Source: CAD feature listing. Evaluate the final solid. Frame: model axes, mm. A direction names the side the tool comes from. Give positions to 0.01 mm unless a question says otherwise; leave off trailing zeros. Write each loop counter-clockwise with the first axis right and the second up, starting at its lowest first coordinate (ties: lowest second). Pieces come first, ordered by that corner, then holes. Notation, with made-up numbers: (14.5, 40.25) -> (25.5, 40.25) arc R25 ccw to (25.5, 63.25) -> close; hole circle Ø1 at (47, 64.25). An arc over 180 degrees is marked (long way). Write item = value, one per line.
from build123d import *

# Parameters (mm, degrees)
F0_W     = 215
F0_H     = 50
F1_DEPTH = 57
F3_DEPTH = 18
F4_W     = 26
F4_H     = 3
F5_DEPTH = 10


with BuildPart() as f1:
    # F0 (on Right) → F1 (new body, symmetric)
    with BuildSketch(Plane.YZ):
        with Locations((-107.5, 25)):
            Rectangle(F0_W, F0_H)
    extrude(amount=F1_DEPTH, both=True)

    # F2 (on face) → F3 (cut)
    with BuildSketch(Plane.XZ.offset(215)):
        Polygon((-55, 50), (-55, 6), (-37, 6), (-37, 21), (50, 21), (50, 6), (55, 6), (55, 50), align=None)
    extrude(amount=-F3_DEPTH, mode=Mode.SUBTRACT)

    # F4 (on face) → F5 (cut)
    with BuildSketch(Plane.XY.offset(50)):
        with Locations((22, -168.5)):
            Rectangle(F4_W, F4_H)
        with Locations((22, -172.5)):
            Rectangle(F4_W, F4_H)
        with Locations((22, -176.5)):
            Rectangle(F4_W, F4_H)
        with Locations((22, -180.5)):
            Rectangle(F4_W, F4_H)
        with Locations((22, -184.5)):
            Rectangle(F4_W, F4_H)
        with Locations((-22, -184.5)):
            Rectangle(F4_W, F4_H)
        with Locations((-22, -180.5)):
            Rectangle(F4_W, F4_H)
        with Locations((-22, -176.5)):
            Rectangle(F4_W, F4_H)
        with Locations((-22, -172.5)):
            Rectangle(F4_W, F4_H)
        with Locations((-22, -168.5)):
            Rectangle(F4_W, F4_H)
    extrude(amount=-F5_DEPTH, mode=Mode.SUBTRACT)


solid = f1.part
(1) Section query A-A (z = 29). Return loops of the section in (x, y).
Values follow:
outline = (-57, -215) -> (-55, -215) -> (-55, -197) -> (55, -197) -> (55, -215) -> (57, -215) -> (57, 0) -> (-57, 0) -> close
(2) Section query B-B (x = 0). Return loops of the section in (y, z), plus the area to 3 significant figures.
Values follow:
outline = (-215, 0) -> (0, 0) -> (0, 50) -> (-197, 50) -> (-197, 21) -> (-215, 21) -> close
area = 10,200 mm2
(3) First-contact query: pin 1 (8 mm diameter, centred on x = 18.5, z = 44.5, fed in from -Y); pin 2 (1.5 mm diameter, centred on x = 17.5, y = -176, fed in from +Z). Flat tips, straight axial feed; report the tip coordinate or a pass-through.
Values follow:
pin_1 = -197
pin_2 = 40
(4) Section query C-C (z = 46). Give the number of separate pieces and of enclosed holes in the cut face, plus the area to 4 significant figures.
Values follow:
separate_pieces = 1
enclosed_holes = 10
area = 21,750 mm2
(5) Material intervals for line 1 (Y direction, x = -27, z = 41); line 2 (Z direction, x = 28, y = -199); line 3 (Y direction, x = -40, z = 29), sorted ascending.
Values follow:
line_1 = -197 to -186, -183 to -182, -179 to -178, -175 to -174, -171 to -170, -167 to 0
line_2 = 0 to 21
line_3 = -197 to 0
(6) Section query D-D (x = 23.5). Return loops of the section in (y, z), plus the area to 3 significant figures.
Values follow:
outline = (-215, 0) -> (0, 0) -> (0, 50) -> (-167, 50) -> (-167, 40) -> (-170, 40) -> (-170, 50) -> (-171, 50) -> (-171, 40) -> (-174, 40) -> (-174, 50) -> (-175, 50) -> (-175, 40) -> (-178, 40) -> (-178, 50) -> (-179, 50) -> (-179, 40) -> (-182, 40) -> (-182, 50) -> (-183, 50) -> (-183, 40) -> (-186, 40) -> (-186, 50) -> (-197, 50) -> (-197, 21) -> (-215, 21) -> close
area = 10,100 mm2
(7) Pull-direction query (Y, two-part tool) for faces 3 (the face through (-57, -109, 25)), 4 (the face through (22, -174, 45)), 5 (the face through (1, 0, 25)); classes: pulls with the +Y half, pulls with the -Y half, needs draft (parallel to the pull), parting line crosses it, or undercut.
Values follow:
face_3 = needs draft
face_4 = undercut
face_5 = pulls with the +Y half
(8) Access query for faces 1 (the face through (55, -206, 28)), 2 (the face through (-22, -174, 45)). Directions: +Z, -Z, +X, -X, +Y, -Y. A direction counts if a zero-diameter tool reaches every point of the face in a straight line with its end or side. Return the directions, or none.
Values follow:
face_1 = +Z, -Y
face_2 = +Z
